Check sheet for the modelled part. Datum: model origin and axes. Units: mm. A direction names the side the tool comes from. Round coordinates to 2 decimals unless told otherwise and drop trailing zeros. Order: outer loops, then holes, each group sorted by start corner. A loop starts at its lowest first (then second) coordinate and runs counter-clockwise, first axis right, second up. Notation, with made-up numbers: (-2, 50.25) -> (19, 50.25) arc R21 ccw to (19, 72.25) -> close; hole circle Ø1 at (-18.75, 65). An arc over 180 degrees is marked (long way). Use CSV: the item, a comma, the result in double quotes.
```python
from build123d import *

# Parameters (mm, degrees)
SKETCH7_R            = 15
BOSS_EXTRUDE2_DEPTH  = 12
SKETCH8_R            = 2.2
CUT_EXTRUDE2_DEPTH   = 20
CUT_EXTRUDE2_DRAFT   = 20
BOSS_EXTRUDE4_START  = -3
SKETCH11_W           = 5
SKETCH11_H           = 10
BOSS_EXTRUDE4_DEPTH  = 48
SKETCH14_W           = 5
SKETCH14_H           = 10
BOSS_EXTRUDE5_DEPTH  = 6.3
SKETCH17_W           = 2.5
SKETCH17_H           = 10
BOSS_EXTRUDE8_DEPTH  = 16
SKETCH20_R           = 1.5
CUT_EXTRUDE3_DEPTH   = 15
FILLET2_R            = 2
FILLET7_R            = 0.5
FILLET8_R            = 0.5
SKETCH24_W           = 3
SKETCH24_H           = 10
BOSS_EXTRUDE11_DEPTH = 7
FILLET2_OF_MIRROR5_R = 2
FILLET9_R            = 0.2
FILLET10_START       = -6
FILLET10_DEPTH       = 12
FILLET10_START_2     = -4.929582237
FILLET10_2_DEPTH     = 10
FILLET11_R           = 0.5


with BuildPart() as part:
    # Sketch7 → Boss-Extrude2 (new body)
    with BuildSketch(Plane.XY.offset(37)):
        Circle(SKETCH7_R)
    extrude(amount=-BOSS_EXTRUDE2_DEPTH)


with BuildPart() as cut_extrude2_tool:
    # Sketch8 → Cut-Extrude2 (with draft: the straight prism first)
    with BuildSketch(Plane.XY.offset(37)):
        Circle(SKETCH8_R)
    extrude(amount=-CUT_EXTRUDE2_DEPTH)
    # Cut-Extrude2: the draft: its side faces are tilted about the plane it starts from
    cut_extrude2_sides = [cut_extrude2_tool.faces().sort_by_distance(p)[0] for p in [
        (-2.2, 0, 27),
    ]]
    draft(cut_extrude2_sides, Plane.XY.offset(37), CUT_EXTRUDE2_DRAFT)


with BuildPart() as part_1:
    add(part.part)

    # Cut-Extrude2: cut by cut_extrude2_tool
    add(cut_extrude2_tool.part, mode=Mode.SUBTRACT)

    # Sketch11 → Boss-Extrude4 (add)
    with BuildSketch(Plane(origin=(15, 0, 0), x_dir=(0, 0, -1), z_dir=(1, 0, 0)).offset(BOSS_EXTRUDE4_START)):
        with Locations((-31.203319291, 0.070417763)):
            Rectangle(SKETCH11_W, SKETCH11_H)
    boss_extrude4 = extrude(amount=BOSS_EXTRUDE4_DEPTH)

    # Sketch14 → Boss-Extrude5 (add)
    with BuildSketch(Plane.XY.offset(33.703319291)):
        with Locations((57.5, 0.070417763)):
            Rectangle(SKETCH14_W, SKETCH14_H)
    boss_extrude5 = extrude(amount=BOSS_EXTRUDE5_DEPTH)

    # Sketch17 → Boss-Extrude8 (add)
    with BuildSketch(Plane.XY.offset(40.003319291)):
        with Locations((56.25, 0.070417763)):
            Rectangle(SKETCH17_W, SKETCH17_H)
    boss_extrude8 = extrude(amount=BOSS_EXTRUDE8_DEPTH)

    # Sketch20 → Cut-Extrude3 (cut)
    with BuildSketch(Plane(origin=(57.5, 0, 0), x_dir=(0, 0, -1), z_dir=(1, 0, 0))):
        with Locations((-42.003319291, 0)):
            Circle(SKETCH20_R)
        with Locations((-48.003319291, 0)):
            Circle(SKETCH20_R)
    cut_extrude3 = extrude(amount=-CUT_EXTRUDE3_DEPTH, mode=Mode.SUBTRACT)

    # Fillet2
    fillet2_edges = [part_1.edges().sort_by_distance(p)[0] for p in [
        (14.166835178, -4.929582237, 31.203319291),
        (14.777611852, 2.573361217, 28.703319291),
        (14.117041606, 5.070417763, 31.203319291),
        (14.777611852, 2.573361217, 33.703319291),
    ]]
    fillet(fillet2_edges, radius=FILLET2_R)

    # Fillet7
    fillet7_edges = [part_1.edges().sort_by_distance(p)[0] for p in [
        (-15, 0, 37),
    ]]
    fillet(fillet7_edges, radius=FILLET7_R)

    # Fillet8
    fillet8_edges = [part_1.edges().sort_by_distance(p)[0] for p in [
        (-15, 0, 25),
    ]]
    fillet(fillet8_edges, radius=FILLET8_R)

    # Sketch24 → Boss-Extrude11 (add)
    with BuildSketch(Plane.ZY.offset(-55)):
        with Locations((51.303319291, 0.070417763)):
            Rectangle(SKETCH24_W, SKETCH24_H)
    boss_extrude11 = extrude(amount=BOSS_EXTRUDE11_DEPTH)

    # Mirror5: Boss-Extrude4, Boss-Extrude5, Boss-Extrude8, Cut-Extrude3, Boss-Extrude11 across plane
    add(boss_extrude4.mirror(Plane(origin=(0, 0, 0), x_dir=(0, 0, 1), z_dir=(1, 0, 0))))
    add(boss_extrude5.mirror(Plane(origin=(0, 0, 0), x_dir=(0, 0, 1), z_dir=(1, 0, 0))))
    add(boss_extrude8.mirror(Plane(origin=(0, 0, 0), x_dir=(0, 0, 1), z_dir=(1, 0, 0))))
    add(cut_extrude3.mirror(Plane(origin=(0, 0, 0), x_dir=(0, 0, 1), z_dir=(1, 0, 0))), mode=Mode.SUBTRACT)
    add(boss_extrude11.mirror(Plane(origin=(0, 0, 0), x_dir=(0, 0, 1), z_dir=(1, 0, 0))))

    # Fillet2 of Mirror5
    fillet2_of_mirror5_edges = [part_1.edges().sort_by_distance(p)[0] for p in [
        (-14.166835178, -4.929582237, 31.203319291),
        (-14.777611852, 2.573361217, 28.703319291),
        (-14.117041606, 5.070417763, 31.203319291),
        (-14.777611852, 2.573361217, 33.703319291),
    ]]
    fillet(fillet2_of_mirror5_edges, radius=FILLET2_OF_MIRROR5_R)

    # Fillet9
    fillet9_edges = [part_1.edges().sort_by_distance(p)[0] for p in [
        (55, 0.070417763, 52.803319291),
        (55, 0.070417763, 49.803319291),
    ]]
    fillet(fillet9_edges, radius=FILLET9_R)

    # Fillet10: read off the stored shape, not the designer's step
    # Fillet10 outline → Fillet10 (cut)
    with BuildSketch(Plane(origin=(0, 0, 0), x_dir=(1, 0, 0), z_dir=(0, 1, 0)).offset(FILLET10_START)):
        with BuildLine():
            Line((48, -49.803319291), (48, -50.303319291))
            ThreePointArc((48, -50.303319291), (48.14644661, -49.949765901), (48.5, -49.803319291))
            Line((48.5, -49.803319291), (48, -49.803319291))
        make_face()
    extrude(amount=FILLET10_DEPTH, mode=Mode.SUBTRACT)

    # Fillet10 2 outline → Fillet10 2 (add)
    with BuildSketch(Plane(origin=(0, 0, 0), x_dir=(1, 0, 0), z_dir=(0, 1, 0)).offset(FILLET10_START_2)):
        with BuildLine():
            ThreePointArc((57.5, -40.503319291), (57.64644661, -40.149765901), (58, -40.003319291))
            Line((58, -40.003319291), (57.5, -40.003319291))
            Line((57.5, -40.003319291), (57.5, -40.503319291))
        make_face()
    extrude(amount=FILLET10_2_DEPTH)

    # Fillet11
    fillet11_edges = [part_1.edges().sort_by_distance(p)[0] for p in [
        (48, 0.070417763, 52.803319291),
    ]]
    fillet(fillet11_edges, radius=FILLET11_R)


solid = part_1.part
```
Q1. Scan lines: L1, parallel to Z at x = -56.65, y = 0; L2, parallel to X at y = -1, z = 44; L3, parallel to Z at x = 30, y = -0.5. Record each from-to range of solid material in increasing order.
Result sheet:
L1,"z = 28.7 to 40.5, 43.5 to 46.5, 49.5 to 56"
L2,"x = -57.5 to -55, 55 to 57.5"
L3,"z = 28.7 to 33.7"
Q2. Access from +Z, -Z, +X, -X, +Y, -Y to the whole of each face (thin tool, end or side, straight path). Record for faces 5 (the face through (-35, 0, 33.703)), 6 (the face through (-38, 0, 28.703)), 7 (the face through (48, 0, 51)), 8 (the face through (-44, 5.07, 33)), 9 (the face through (59, 0, 40.003)).
Result sheet:
face 5,"+Y, -Y"
face 6,"-Z, -X, +Y, -Y"
face 7,"+Z, +Y, -Y"
face 8,"+Z, -Z, -X, +Y"
face 9,"+Z, +X, +Y, -Y"
Q3. Mould release check, pull along Z, two halves, no side actions. Record for faces 1 (the face through (38, 0, 28.703)), 2 (the face through (-48, 0, 51)), 3 (the face through (-55, 0, 40)), 4 (the face through (52, 0, 49.803)): pulls with the +Z half, pulls with the -Z half, needs draft (parallel to the pull), parting line crosses it, or undercut.
Result sheet:
face 1,"pulls with the -Z half"
face 2,"needs draft"
face 3,"undercut"
face 4,"undercut"
Q4. Sectioned sample at C-C, the plane x = 31.5. Enter the section's corners in (y, z).
Result sheet:
outline,"(-4.93, 28.7) -> (5.07, 28.7) -> (5.07, 33.7) -> (-4.93, 33.7) -> close"
Q5. Sectioned sample at B-B, the plane z = 30. Enter the section's corners in (x, y).
Result sheet:
outline,"(-60, -4.93) -> (-15.52, -4.93) arc R2 cw to (-13.7, -6.11) arc R15 ccw to (13.7, -6.11) arc R2 cw to (15.52, -4.93) -> (60, -4.93) -> (60, 5.07) -> (15.46, 5.07) arc R2 cw to (13.64, 6.24) arc R15 ccw to (-13.64, 6.24) arc R2 cw to (-15.46, 5.07) -> (-60, 5.07) -> close; hole circle Ø9.5 at (0, 0)"
Q6. Sectioned sample at A-A, the plane x = 0. Enter the section's corners in (y, z).
Result sheet:
outline,"(-15, 25.5) arc R0.5 ccw to (-14.5, 25) -> (-6.57, 25) -> (-2.2, 37) -> (-14.5, 37) arc R0.5 ccw to (-15, 36.5) -> close; (2.2, 37) -> (6.57, 25) -> (14.5, 25) arc R0.5 ccw to (15, 25.5) -> (15, 36.5) arc R0.5 ccw to (14.5, 37) -> close"
Q7. Go/stop test with flat-tipped pins: pin 1 (2.5 mm diameter, centred on y = -0.5, z = 55, fed in from +X); pin 2 (5 mm diameter, centred on y = -7.5, z = 49, fed in from -X); pin 3 (8 mm diameter, centred on x = -26.5, y = 2, fed in from +Z); pin 4 (5 mm diameter, centred on y = 0, z = 48, fed in from -X). Record where each tip stops, or that it passes through.
Result sheet:
pin 1,"stops at x = 57.5"
pin 2,"passes through"
pin 3,"stops at z = 33.7"
pin 4,"stops at x = -57.5"
